Here's the drawing with two shaded views (mm, measured from the low corner). I have some questions. A direction names the side the tool comes from. Round coordinates to 2 decimals unless told otherwise and drop trailing zeros. Loops run counter-clockwise (first coordinate to the right, second up) from the corner with the lowest first, then second, coordinate; pieces in that order, holes last. Notation, with made-up numbers: M -7,81.25 L 1,81.25 A34 cw 1,113.25 Z; hole C -3.5,82.25 d3. An arc over 180 degrees is marked long. Answer as a JSON object with one key per item and string values.
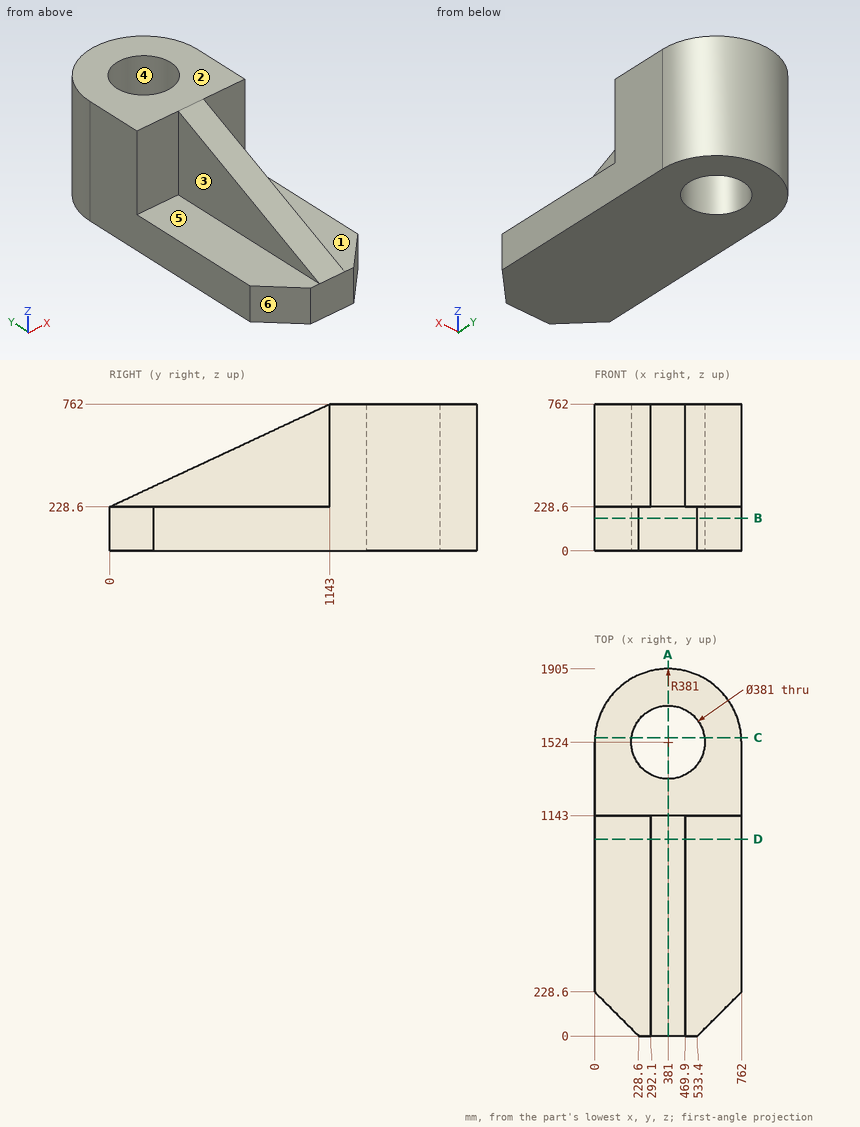
Item 1: I want a section at B-B on z = 170. List the corners of the cut face in (x, y) for me, plus the area to 3 significant figures.
Solution:
{"outline": "M 0,228.6 L 228.6,0 L 533.4,0 L 762,228.6 L 762,1524 A381 ccw 0,1524 Z; hole C 381,1524 d381", "area": "1,220,000 mm2"}
Item 2: I want a section at D-D on y = 1021.5. List the corners of the cut face in (x, z) for me, plus the area to 3 significant figures.
Solution:
{"outline": "M 0,0 L 762,0 L 762,228.6 L 469.9,228.6 L 469.9,705.3 L 292.1,705.3 L 292.1,228.6 L 0,228.6 Z", "area": "259,000 mm2"}
Item 3: For the marked faces 1, 2 and 3, which set-ups out of +Z, -Z, +X, -X, +Y, -Y let a thin tool reach every point of the face, with its end or its side?
Solution:
{"face 1": "+Z, +X, -Y", "face 2": "+Z, +X, -X, +Y, -Y", "face 3": "+Z, -X, -Y"}
Item 4: If I drill on L1, parallel to Z at x = 270, y = 313; L2, parallel to Y at x = 381, z = 379; L3, parallel to X at y = 1056.5, z = 577, over which ranges is the centre line in solid material (lowest first)? Write a range as from..to.
Solution:
{"L1": "z = 0..228.6", "L2": "y = 322.29..1333.5, 1714.5..1905", "L3": "x = 292.1..469.9"}
Item 5: I want a section at A-A on x = 381. List the corners of the cut face in (y, z) for me.
Solution:
{"outline": "M 0,0 L 1333.5,0 L 1333.5,762 L 1143,762 L 0,228.6 Z; M 1714.5,0 L 1905,0 L 1905,762 L 1714.5,762 Z"}
Item 6: We'd pull the mould along X, two halves only. Please class the marked faces 4, 5 and 6: +X half, -X half, draft (parallel to the pull), parting line (faces both ways), or undercut.
Solution:
{"face 4": "undercut", "face 5": "draft", "face 6": "-X half"}
Item 7: I want a section at C-C on y = 1548. List the corners of the cut face in (x, z) for me, plus the area to 3 significant figures.
Solution:
{"outline": "M 0.76,0 L 192.02,0 L 192.02,762 L 0.76,762 Z; M 569.98,0 L 761.24,0 L 761.24,762 L 569.98,762 Z", "area": "291,000 mm2"}
Item 8: For P1, Ø8, axis at y = 261.5, z = 145.5, coming from the -X side; P2, Ø3, axis at x = 623.5, z = 442, coming from the +Y side; P3, Ø10, axis at y = 638.5, z = 458.5, coming from the +X side, each with a flat end and sliding along its axis, tell me the tip position at first contact or that it passes through.
Solution:
{"P1": "stops at x = 0", "P2": "stops at y = 1819.09", "P3": "stops at x = 469.9"}
